Here's how the part is built. I have some questions about the finished solid (model axes, mm). A direction names the side the tool comes from. Round coordinates to 2 decimals unless told otherwise and drop trailing zeros. Write each loop counter-clockwise with the first axis right and the second up, starting at its lowest first coordinate (ties: lowest second). Pieces come first, ordered by that corner, then holes. Notation, with made-up numbers: (-16.5, 74) - (42.5, 74) arc R34 ccw to (42.5, 111) - close; hole circle Ø5 at (-27.5, -29). An arc over 180 degrees is marked (long way). Write item = value, one per line. Start each with the question number.
Item 1: If we section it at C-C (y = -21.75): Please give me the cut outline in (x, z), and give its area (3 significant figures).
Item 2: For P1, Ø1.9, axis at x = 8.5, z = 37.5, coming from the +Y side; P2, Ø3, axis at x = 34.5, y = -8, coming from the -Z side; P3, Ø3, axis at y = -11.5, z = 29.5, coming from the +X side; P4, Ø5, axis at y = -19, z = -22.5, coming from the +X side, each with a flat end and sliding along its axis, tell me the tip position at first contact or that it passes through.
Item 3: If I drill on line 1 along X through (y, z) = (-13, -17); line 2 along Y through (x, z) = (6.5, -26.5) (3 decimals); line 3 along Z through (x, y) = (14, -12.75), over which ranges is the centre line in solid material (lowest first)? Write a range as [from, to].
Item 4: If we section it at A-A (z = -3.5): Please give me the cut outline in (x, y) (3 decimals).
Item 5: If we section it at D-D (z = -27): Please give me the cut outline in (x, y) (3 decimals).
Item 6: If we section it at B-B (y = -14): Please give me the cut outline in (x, z).
Item 7: Thinking about a two-plate mould opening in Y: for faces 1 (the face through (16, 0, 4)), 2 (the face through (41.612, -13, 1)), 3 (the face through (16.27, -10.942, 15.603)), 4 (the face through (16, -25.4, 4)), which applies, pulls with the +Y half, pulls with the -Y half, needs draft (parallel to the pull), parting line crosses it, or undercut?
Item 8: Which directions (+Z, -Z, +X, -X, +Y, -Y) give clear straight access to the entire face, cutting with the end or side of a thin tool? Please do faces 5 (the face through (6.212, -13, -15)), 6 (the face through (0, -18, 4)).
```python
from build123d import *

# Parameters (mm, degrees)
F1_DEPTH = 25.4
F2_R     = 3.81
F3_DEPTH = 69.8653654545
F4_W     = 3.175
F4_H     = 3.175
F5_DEPTH = 84.483178092


with BuildPart() as f1:
    # F0 (on Front) → F1 (new body)
    with BuildSketch(Plane.XZ):
        Polygon((0, 45.3323423862), (0, 0), (0, -39.1498357058), (16.7319830507, -39.1498357058), (41.6124537587, -17.4258463085), (41.6124537587, 19.3378273398), (18.7744107097, 45.3323423862), align=None)
    extrude(amount=F1_DEPTH)

    # F2 (on face) → F3 (cut, through all)
    with BuildSketch(Plane(origin=(33.0732626697, 0, 29.057229776), x_dir=(0, 1, 0), z_dir=(0.7512454532, 0, 0.6600229306))):
        with Locations((-12.7, 4.3632278543)):
            Circle(F2_R)
    extrude(amount=-F3_DEPTH, mode=Mode.SUBTRACT)

    # F4 (on face) → F5 (cut, through all)
    with BuildSketch(Plane.XY.offset(45.3323423862)):
        with Locations((7.7997053549, -14.2875)):
            Rectangle(F4_W, F4_H)
        with Locations((7.7997053549, -11.1125)):
            Rectangle(F4_W, F4_H)
        with Locations((10.9747053549, -11.1125)):
            Rectangle(F4_W, F4_H)
        with Locations((10.9747053549, -14.2875)):
            Rectangle(F4_W, F4_H)
    extrude(amount=-F5_DEPTH, mode=Mode.SUBTRACT)


solid = f1.part
```
Reply:
q1.outline = (0, -39.15) - (16.73, -39.15) - (41.61, -17.43) - (41.61, 19.34) - (18.77, 45.33) - (0, 45.33) - close
q1.area = 2,950 mm2
q2.P1 = 0
q2.P2 = -24.95
q2.P3 = 34
q2.P4 = 38.66
q3.line_1 = [0, 6.21], [12.56, 41.61]
q3.line_2 = [-25.4, -15.875], [-9.525, 0]
q3.line_3 = [-39.15, 13.04], [23.18, 45.33]
q4.outline = (0, -25.4) - (41.612, -25.4) - (41.612, 0) - (0, 0) - close; hole (6.212, -15.875) - (12.562, -15.875) - (12.562, -9.525) - (6.212, -9.525) - close
q5.outline = (0, -25.4) - (30.647, -25.4) - (30.647, 0) - (0, 0) - close; hole (6.212, -15.875) - (12.562, -15.875) - (12.562, -9.525) - (6.212, -9.525) - close
q6.outline = (0, -39.15) - (6.21, -39.15) - (6.21, 6.5) - (0, 1.04) - close; (0, 10.58) - (6.21, 16.03) - (6.21, 45.33) - (0, 45.33) - close; (12.56, -39.15) - (16.73, -39.15) - (41.61, -17.43) - (41.61, 19.34) - (32.56, 29.64) - (12.56, 12.08) - close; (12.56, 21.61) - (27.83, 35.03) - (18.77, 45.33) - (12.56, 45.33) - close
q7.face_1 = pulls with the +Y half
q7.face_2 = needs draft
q7.face_3 = undercut
q7.face_4 = pulls with the -Y half
q8.face_5 = +Z, -Z
q8.face_6 = +Z, -Z, -X, +Y, -Y
